Verification items for the finished model (mm, model axes). A direction names the side the tool comes from. Give positions to 0.01 mm unless a question says otherwise; leave off trailing zeros. Order: outer loops, then holes, each group sorted by start corner. A loop starts at its lowest first (then second) coordinate and runs counter-clockwise, first axis right, second up. Notation, with made-up numbers: M -18,81.25 L 13,81.25 A25 ccw 13,94.25 Z; hole C 55,-1.75 d8. An arc over 180 degrees is marked long. Answer as a JSON object with one key per item and string values.
```python
from build123d import *

# Parameters (mm, degrees)
F0_R     = 2
F1_DEPTH = 75
F2_W     = 10
F2_H     = 75
F3_DEPTH = 5
F4_W     = 2.5
F4_H     = 75
F5_DEPTH = 5
F7_DEPTH = 5
F9_DEPTH = 5


with BuildPart() as f1:
    # F0 (on Top) → F1 (new body)
    with BuildSketch(Plane.XY):
        with BuildLine():
            Line((75, 0.6), (-0.3646306216, 16.9319457282))
            ThreePointArc((-0.3646306216, 16.9319457282), (-3.9741969781, 13.6073776176), (0.3744351102, 11.3333676429))
            ThreePointArc((0.3744351102, 11.3333676429), (1.3807008009, 12.1745510972), (1.9319457282, 13.3646306216))
            Line((1.9319457282, 13.3646306216), (63.6037432565, 0))
            Line((63.6037432565, 0), (75, 0))
            Line((75, 0), (76.2, 0))
            Line((76.2, 0), (125, 0))
            Line((125, 0), (126.2, 0))
            Line((126.2, 0), (125, 0.6))
            Line((125, 0.6), (75, 0.6))
        make_face()
        with Locations((-1, 14)):
            Circle(F0_R, mode=Mode.SUBTRACT)
    extrude(amount=F1_DEPTH)

    # F2 (on face) → F3 (join)
    with BuildSketch(Plane(origin=(2.8529405822, 13.1650457786, 0), x_dir=(0.9773152427, -0.2117897928, 0), z_dir=(-0.2117897928, -0.9773152427, 0))):
        with Locations((4.0576276581, 37.5)):
            Rectangle(F2_W, F2_H)
    extrude(amount=F3_DEPTH)

    # F4 (on face) → F5 (cut)
    with BuildSketch(Plane(origin=(8.8521575732, -1.9183130849, 0), x_dir=(0.2117897928, 0.9773152427, 0), z_dir=(0.9773152427, -0.2117897928, 0))):
        with Locations((12.2206236054, 37.5)):
            Rectangle(F4_W, F4_H)
    extrude(amount=-F5_DEPTH, mode=Mode.SUBTRACT)

    # F6 (on face) → F7 (cut)
    with BuildSketch(Plane.XY.offset(75)):
        Polygon((6.2890474598, 9.8623935508), (6.8185219418, 12.3056816576), (1.9319457282, 13.3646306216), (0.8729967642, 8.478054408), (10.6461491915, 6.36015648), (11.1756236735, 8.8034445868), align=None)
    extrude(amount=-F7_DEPTH, mode=Mode.SUBTRACT)

    # F8 (on face) → F9 (cut)
    with BuildSketch(Plane(origin=(0, 0, 0), x_dir=(1, 0, 0), z_dir=(0, 0, -1))):
        Polygon((1.9319457282, -13.3646306216), (6.8185219418, -12.3056816576), (6.2890474598, -9.8623935508), (11.1756236735, -8.8034445868), (10.6461491915, -6.36015648), (0.8729967642, -8.478054408), align=None)
    extrude(amount=-F9_DEPTH, mode=Mode.SUBTRACT)


solid = f1.part
```
Q1. Section check B-B on x = 93. Record the cut outline in (y, z).
Resolved:
{"outline": "M 0,0 L 0.6,0 L 0.6,75 L 0,75 Z"}
Q2. Gauge pin test, flat ends, axial feed: pin 1 Ø4 at (x, z) = (15, 32) entering from -Y; pin 2 Ø3.5 at (x, y) = (7.5, 8.5) entering from +Z; pin 3 Ø1 at (x, z) = (19, 25.5) entering from +Y. Record the tip position at first contact, or that the pin passes through.
Resolved:
{"pin 1": "stops at y = 10.1", "pin 2": "stops at z = 70", "pin 3": "stops at y = 12.84"}
Q3. Section check C-C on y = 2.5. Record the cut outline in (x, z).
Resolved:
{"outline": "M 52.07,0 L 66.23,0 L 66.23,75 L 52.07,75 Z"}
Q4. Release check for a two-part mould opening along Y. For faces 5 (the face through (-1, 16, 37)), 6 (the face through (37.85, 8.65, 36.98)), 7 (the face through (6, 10, 70)) record: +Y half, -Y half, draft (parallel to the pull), parting line (faces both ways), or undercut.
Resolved:
{"face 5": "undercut", "face 6": "+Y half", "face 7": "draft"}
Q5. Section check A-A on z = 60.5. Record the cut outline in (x, y), then the cut area to 3 significant figures.
Resolved:
{"outline": "M -0.36,16.93 A3 ccw long 1.93,13.36 L 0.87,8.48 L 10.65,6.36 L 11.18,8.8 L 6.29,9.86 L 6.82,12.31 L 63.6,0 L 126.2,0 L 125,0.6 L 75,0.6 Z; hole C -1,14 d4", "area": "295 mm²"}
Q6. Tool access check on faces 1 (the face through (11, 8, 37)), 2 (the face through (100, 0.6, 37)), 3 (the face through (6, 10, 5)), 4 (the face through (6.55, 11.07, 37.96)). Record the directions out of +Z, -Z, +X, -X, +Y, -Y that give a thin tool (end or side, any length) a straight path to the whole face; none if there is none.
Resolved:
{"face 1": "+Z, -Z, -Y", "face 2": "+Z, -Z, +X, +Y", "face 3": "-Z, -Y", "face 4": "+Z, -Z"}
Q7. Material ranges on L1, parallel to Y at x = -1, z = 59.5; L2, parallel to Y at x = 114, z = 14.5; L3, parallel to Y at x = 18, z = 63, recorded low to high.
Resolved:
{"L1": "y = 11 to 12, 16 to 17", "L2": "y = 0 to 0.6", "L3": "y = 9.88 to 12.95"}
